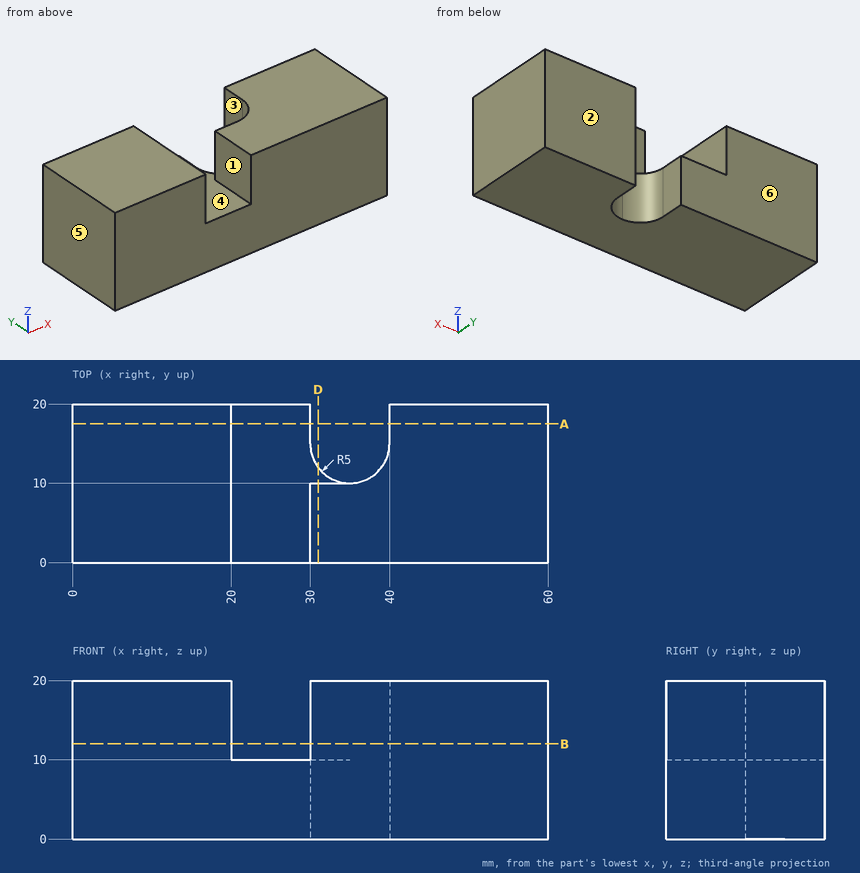
Drawing for the job (mm, zero at the part's lowest x, y, z). A direction names the side the tool comes from. Coordinates: 2 decimals unless noted, no trailing zeros. Write each loop counter-clockwise with the first axis right and the second up, starting at its lowest first coordinate (ties: lowest second). Pieces come first, ordered by that corner, then holes. Notation, with made-up numbers: (11, 51) - (67, 51) arc R19 ccw to (67, 83) - close; hole circle Ø1 at (46, 20). An arc over 180 degrees is marked (long way). Write each question's results on one line, items separated by ' | '. Start each with the question number.
1) Mould opens along X. For the marked faces 4, 5 and 6 say: pulls with the +X half, pulls with the -X half, needs draft (parallel to the pull), parting line crosses it, or undercut.
2) Cut at B-B (z = 12). Write the cut outline in (x, y), then the cut area to 3 significant figures.
3) Probe line 1 along X through (y, z) = (6, 13.75); line 2 along X through (y, z) = (17, 16.75); line 3 along Z through (x, y) = (29, 11). List the from-to ranges inside material, lowest first. Write a range as from..to.
4) Flat gauge pin, fed straight in: P1, Ø2.5, axis at x = 33.5, z = 5.5, coming from the +Y side. Where does the tip first touch, or does it go through?
5) Cut at A-A (y = 17.5). Write the cut outline in (x, z).
6) Cut at D-D (x = 31). Write the cut outline in (y, z), then the cut area to 3 significant figures.
7) 3-axis set-ups, long thin cutter, end or side, ignore diameter. For the marked faces 1, 2 and 3: which of +Z, -Z, +X, -X, +Y, -Y reach the whole face in a straight line?
Returned:
1) face 4: undercut | face 5: pulls with the -X half | face 6: needs draft
2) outline: (0, 0) - (20, 0) - (20, 20) - (0, 20) - close; (30, 0) - (60, 0) - (60, 20) - (40, 20) - (40, 15) arc R5 cw to (35, 10) - (30, 10) - close | area: 905 mm^2
3) line 1: 0..20, 30..60 | line 2: 0..20, 40..60 | line 3: 0..10
4) P1: y = 10.82
5) outline: (0, 0) - (30, 0) - (30, 10) - (20, 10) - (20, 20) - (0, 20) - close; (40, 0) - (60, 0) - (60, 20) - (40, 20) - close
6) outline: (0, 0) - (12, 0) - (12, 10) - (10, 10) - (10, 20) - (0, 20) - close | area: 220 mm^2
7) face 1: +Z, +Y, -Y | face 2: +Z, -Z, +X, -X, +Y | face 3: +Z, -Z, +Y
